Drawing for the job (mm, zero at the part's lowest x, y, z). Coordinates: 2 decimals unless noted, no trailing zeros. Order: outer loops, then holes, each group sorted by start corner. A loop starts at its lowest first (then second) coordinate and runs counter-clockwise, first axis right, second up.
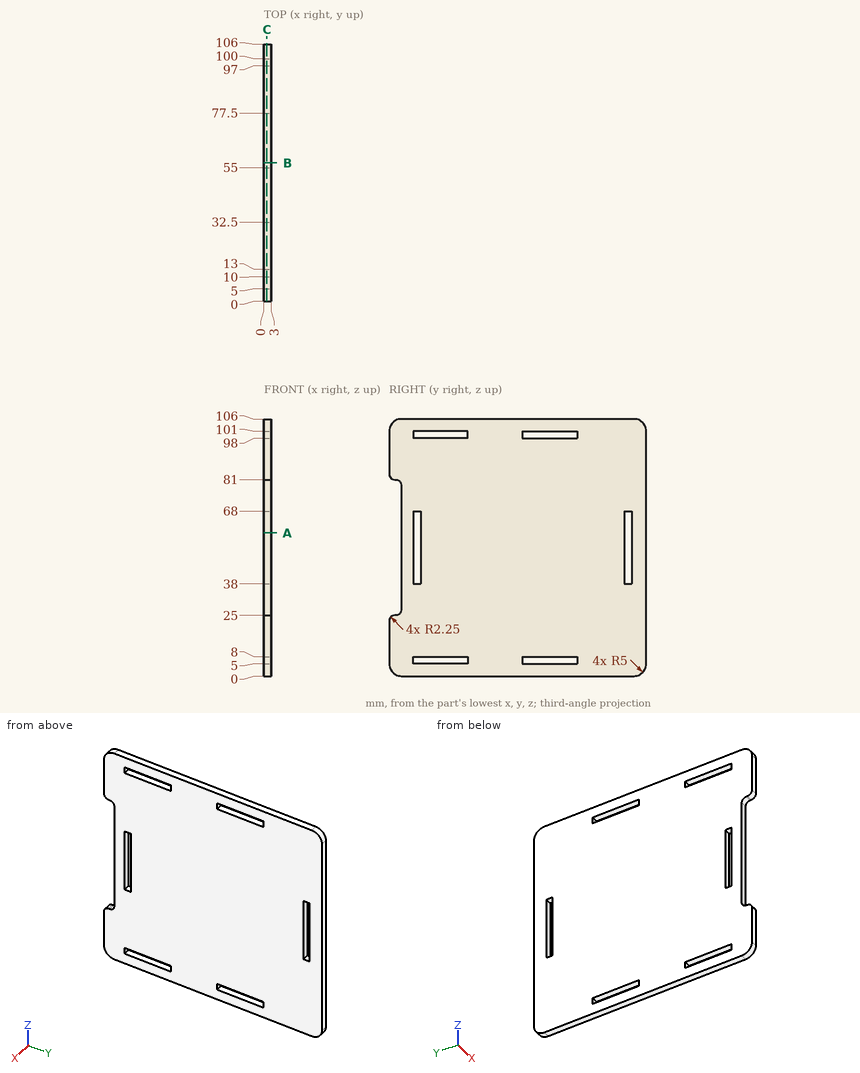
1) Slice it at B-B (y = 57). List the corners of the cut face in (x, z), plus the area to 3 significant figures.
2) Slice it at C-C (x = 1.25). Give the number of separate pieces and of enclosed holes in the cut face, plus the area to 3 significant figures.
3) Slice it at A-A (z = 59). List the corners of the cut face in (x, y).
4) Drill centre lines: probe 1 along Z at (x, y) = (1.3, 60.5); probe 2 along Z at (x, y) = (1.7, 11); probe 3 along Y at (x, z) = (1.5, 49). Where is each one in solid material? Low to high.
5) Pin check, flat tip, straight feed: P1, Ø1.5, axis at x = 2, z = 47.5, coming from the -Y side. Stop position of the tip, or through.
Worked out:
1. outline: (0, 0) - (3, 0) - (3, 5) - (0, 5) - close; (0, 8) - (3, 8) - (3, 98) - (0, 98) - close; (0, 101) - (3, 101) - (3, 106) - (0, 106) - close
1. area: 300 mm2
2. separate pieces: 1
2. enclosed holes: 6
2. area: 10,500 mm2
3. outline: (0, 5) - (3, 5) - (3, 10) - (0, 10) - close; (0, 13) - (3, 13) - (3, 97) - (0, 97) - close; (0, 100) - (3, 100) - (3, 106) - (0, 106) - close
4. probe 1: z = 0 to 5, 8 to 98, 101 to 106
4. probe 2: z = 0 to 5, 8 to 38, 68 to 98, 101 to 106
4. probe 3: y = 5 to 10, 13 to 97, 100 to 106
5. P1: stops at y = 5
